Geometry check sheet. Reference: the model listing, model coordinates, mm. Face numbers are marked on the shaded views. Round coordinates to 2 decimals unless told otherwise and drop trailing zeros. Loops run counter-clockwise (first coordinate to the right, second up) from the corner with the lowest first, then second, coordinate; pieces in that order, holes last. Notation, with made-up numbers: (-33.5, 20) -> (15.5, 20) arc R10 ccw to (15.5, 28) -> close; hole circle Ø10 at (-37.75, 70.5). An arc over 180 degrees is marked (long way). Use a Markdown table: item, result. Add a question column.
Q1. Sectioned sample at C-C, the plane x = 0. Give the number of separate pieces and of enclosed holes in the cut face, then the cut area to 3 significant figures.
Q2. Material ranges on L1, parallel to Z at x = 0, y = 2.75; L2, parallel to X at y = 5.45, z = -17.5; L3, parallel to Z at x = 1, y = 6.25, recorded low to high.
Q3. Sectioned sample at A-A, the plane z = -17.5. Enter the section's corners in (x, y), then the cut area to 3 significant figures.
Q4. Sectioned sample at B-B, the plane y = 6. Enter the section's corners in (x, z).
Q5. Release check for a two-part mould opening along Z. For the marked faces 1, 2 and 3 record: released by +Z, released by -Z, zero draft, split by the parting line, or undercut.
Q6. Sectioned sample at D-D, the plane x = 8. Enter the section's corners in (y, z).
Q7. Gauge pin test, flat ends, axial feed: P1, Ø7.5, axis at x = 0, z = -17.5, coming from the +Y side; P2, Ø16.5, axis at x = 0, z = 0, coming from the +Y side. Record the tip position at first contact, or that the pin passes through.
```python
from build123d import *

# Parameters (mm, degrees)
SKETCH1_W           = 41
SKETCH1_H           = 70
BOSS_EXTRUDE1_DEPTH = 8
FILLET1_R           = 4
CHAMFER1_SIZE       = 1
SKETCH2_R           = 3.3
CUT_EXTRUDE1_DEPTH  = 8
CHAMFER2_SIZE       = 3.2
SKETCH3_R           = 5.5
CUT_EXTRUDE2_DEPTH  = 4.2
SKETCH4_R           = 5.1
CUT_EXTRUDE3_DEPTH  = 10
SKETCH5_R           = 10
CUT_EXTRUDE5_DEPTH  = 4


with BuildPart() as part:
    # Sketch1 → Boss-Extrude1 (new body)
    with BuildSketch(Plane(origin=(0, 0, 0), x_dir=(1, 0, 0), z_dir=(0, 1, 0))):
        Rectangle(SKETCH1_W, SKETCH1_H)
    extrude(amount=BOSS_EXTRUDE1_DEPTH)

    # Fillet1
    fillet1_edges = [part.edges().sort_by_distance(p)[0] for p in [
        (20.5, 4, 35),
        (-20.5, 4, 35),
        (-20.5, 4, -35),
        (20.5, 4, -35),
    ]]
    fillet(fillet1_edges, radius=FILLET1_R)

    # Chamfer1
    chamfer1_edges = [part.edges().sort_by_distance(p)[0] for p in [
        (-20.5, 0, 0),
        (-20.5, 8, 0),
        (20.5, 0, 0),
        (0, 0, 35),
        (0, 0, -35),
        (-19.328427125, 0, 33.828427125),
        (19.328427125, 0, 33.828427125),
        (19.328427125, 0, -33.828427125),
        (-19.328427125, 0, -33.828427125),
        (0, 8, -35),
        (20.5, 8, 0),
        (0, 8, 35),
        (-19.328427125, 8, 33.828427125),
        (19.328427125, 8, 33.828427125),
        (19.328427125, 8, -33.828427125),
        (-19.328427125, 8, -33.828427125),
    ]]
    chamfer(chamfer1_edges, length=CHAMFER1_SIZE)

    # Sketch2 → Cut-Extrude1 (cut)
    with BuildSketch(Plane(origin=(0, 8, 0), x_dir=(1, 0, 0), z_dir=(0, 1, 0))):
        with Locations((0, -17.5)):
            Circle(SKETCH2_R)
        with Locations((0, 17.5)):
            Circle(SKETCH2_R)
    extrude(amount=-CUT_EXTRUDE1_DEPTH, mode=Mode.SUBTRACT)

    # Chamfer2
    chamfer2_edges = [part.edges().sort_by_distance(p)[0] for p in [
        (-3.3, 8, 17.5),
    ]]
    chamfer(chamfer2_edges, length=CHAMFER2_SIZE)

    # Sketch3 → Cut-Extrude2 (cut)
    with BuildSketch(Plane(origin=(0, 8, 0), x_dir=(1, 0, 0), z_dir=(0, 1, 0))):
        with Locations((0, 17.5)):
            Circle(SKETCH3_R)
    extrude(amount=-CUT_EXTRUDE2_DEPTH, mode=Mode.SUBTRACT)

    # Sketch4 → Cut-Extrude3 (cut)
    with BuildSketch(Plane(origin=(0, 8, 0), x_dir=(1, 0, 0), z_dir=(0, 1, 0))):
        Circle(SKETCH4_R)
    extrude(amount=-CUT_EXTRUDE3_DEPTH, mode=Mode.SUBTRACT)

    # Sketch5 → Cut-Extrude5 (cut)
    with BuildSketch(Plane(origin=(0, 8, 0), x_dir=(1, 0, 0), z_dir=(0, 1, 0))):
        Circle(SKETCH5_R)
    extrude(amount=-CUT_EXTRUDE5_DEPTH, mode=Mode.SUBTRACT)


solid = part.part
```
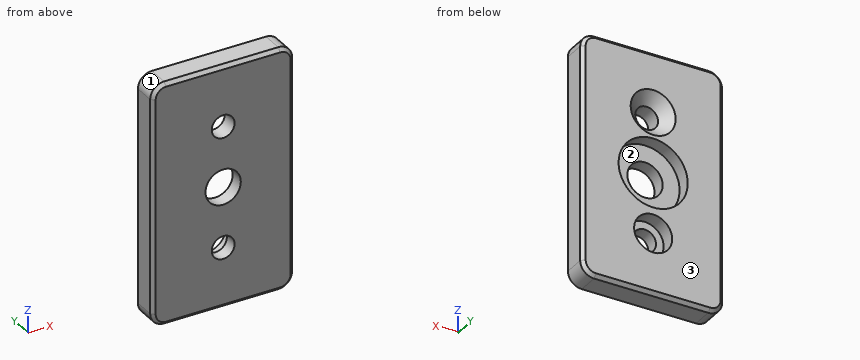
Values:
| question | item | result |
|---|---|---|
| 1 | separate pieces | 4 |
| 1 | enclosed holes | 0 |
| 1 | area | 303 mm^2 |
| 2 | L1 | -35 to -20.8, -14.2 to -5.1, 5.1 to 14.2, 20.8 to 35 |
| 2 | L2 | -20.5 to -5.5, 5.5 to 20.5 |
| 2 | L3 | -35 to -22.91, -12.09 to -9.95, 9.95 to 12.86, 22.14 to 35 |
| 3 | outline | (-20.5, 1) -> (-19.5, 0) -> (-3.3, 0) -> (-3.3, 3.8) -> (-5.5, 3.8) -> (-5.5, 8) -> (-19.5, 8) -> (-20.5, 7) -> close; (3.3, 0) -> (19.5, 0) -> (20.5, 1) -> (20.5, 7) -> (19.5, 8) -> (5.5, 8) -> (5.5, 3.8) -> (3.3, 3.8) -> close |
| 3 | area | 255 mm^2 |
| 4 | outline | (-20.5, -31) arc R4 ccw to (-16.5, -35) -> (16.5, -35) arc R4 ccw to (20.5, -31) -> (20.5, 31) arc R4 ccw to (16.5, 35) -> (-16.5, 35) arc R4 ccw to (-20.5, 31) -> close; hole circle Ø20 at (0, 0); hole circle Ø11 at (0, -17.5); hole circle Ø9 at (0, 17.5) |
| 5 | face 1 | released by +Z |
| 5 | face 2 | undercut |
| 5 | face 3 | zero draft |
| 6 | outline | (0, -34) -> (1, -35) -> (7, -35) -> (8, -34) -> (8, -6) -> (4, -6) -> (4, 6) -> (8, 6) -> (8, 34) -> (7, 35) -> (1, 35) -> (0, 34) -> close |
| 7 | P1 | y = 3.8 |
| 7 | P2 | y = 4 |
